Here's the drawing with two shaded views (mm, measured from the low corner). I have some questions. A direction names the side the tool comes from. Give positions to 0.01 mm unless a question says otherwise; leave off trailing zeros. Loops run counter-clockwise (first coordinate to the right, second up) from the corner with the lowest first, then second, coordinate; pieces in that order, holes last. Notation, with made-up numbers: (-40, 64) -> (-17, 64) arc R21 cw to (-17, 90) -> close; hole circle Ø10 at (72.5, 51.25). An arc over 180 degrees is marked (long way). Answer in a Markdown table with one row per item. Add a question column.
Item 1: Which directions (+Z, -Z, +X, -X, +Y, -Y) give clear straight access to the entire face, cutting with the end or side of a thin tool? Please do the marked faces 1 and 2.
Item 2: If we section it at B-B (z = 40.5): Write out the boundary of the cut face in (x, y) (1 decimal).
Item 3: If I drill on line 1 (Y direction, x = 1.1, z = 40.5); line 2 (Y direction, x = 5.25, z = 3) (1 decimal); line 3 (Z direction, x = 3, y = 6) (1 decimal), over which ranges is the centre line in solid material (lowest first)?
Item 4: If we section it at A-A (y = 6.35): Write out the boundary of the cut face in (x, z) (1 decimal), then the cut area to 3 significant figures.
Item 5: For P1, Ø7.5, axis at x = 9.5, z = 36, coming from the +Y side (3 decimals), with a flat end and sliding along its axis, tell me the tip position at first contact or that it passes through.
Item 6: If we section it at C-C (y = 11.5): Write out the boundary of the cut face in (x, z) (1 decimal).
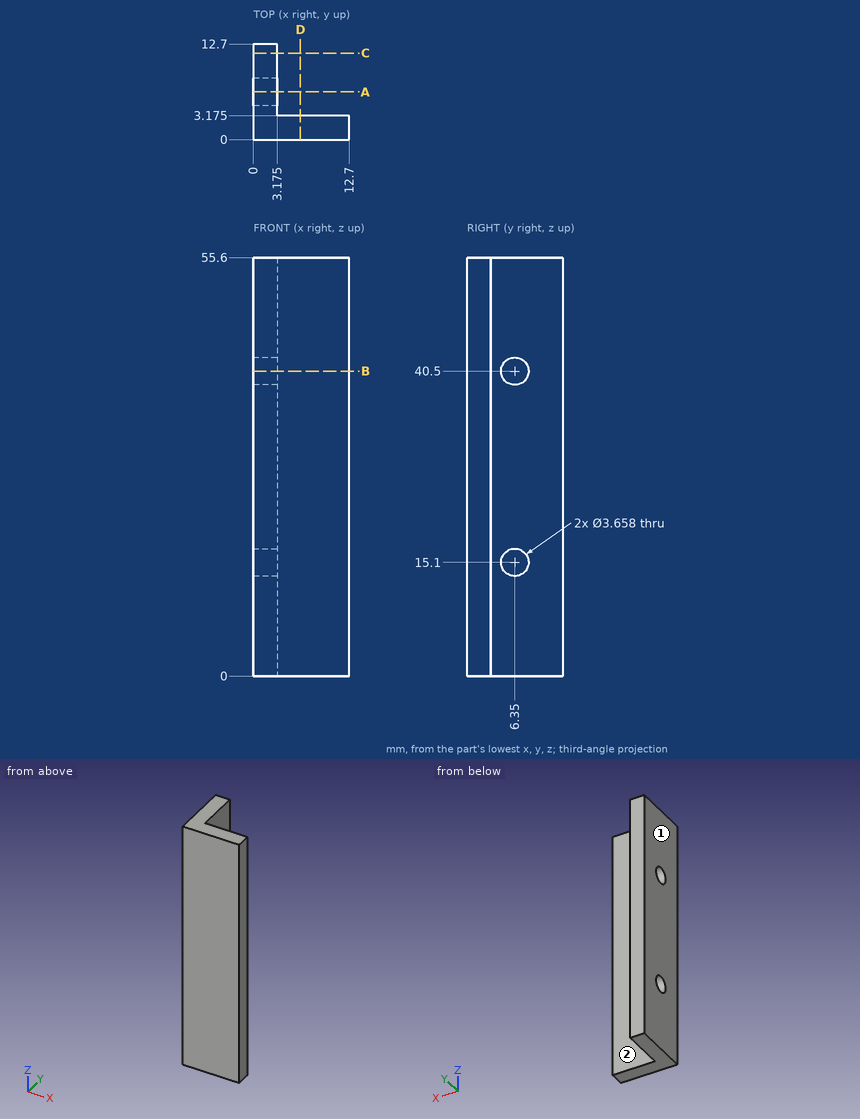
Recorded:
| question | item | result |
|---|---|---|
| 1 | face 1 | +Z, -Z, -X, +Y, -Y |
| 1 | face 2 | +Z, -Z, +X, +Y |
| 2 | outline | (0, 0) -> (12.7, 0) -> (12.7, 3.2) -> (3.2, 3.2) -> (3.2, 4.5) -> (0, 4.5) -> close; (0, 8.2) -> (3.2, 8.2) -> (3.2, 12.7) -> (0, 12.7) -> close |
| 3 | line 1 | y = 0 to 4.52, 8.18 to 12.7 |
| 3 | line 2 | y = 0 to 3.2 |
| 3 | line 3 | z = 0 to 13.3, 16.9 to 38.7, 42.3 to 55.6 |
| 4 | outline | (0, 0) -> (3.2, 0) -> (3.2, 13.3) -> (0, 13.3) -> close; (0, 16.9) -> (3.2, 16.9) -> (3.2, 38.7) -> (0, 38.7) -> close; (0, 42.3) -> (3.2, 42.3) -> (3.2, 55.6) -> (0, 55.6) -> close |
| 4 | area | 153 mm^2 |
| 5 | P1 | stops at y = 3.175 |
| 6 | outline | (0, 0) -> (3.2, 0) -> (3.2, 55.6) -> (0, 55.6) -> close |
